Build history of the part. All positions in model axes, mm. A direction names the side the tool comes from. Coordinates: 2 decimals unless noted, no trailing zeros. Loops run counter-clockwise (first coordinate to the right, second up) from the corner with the lowest first, then second, coordinate; pieces in that order, holes last.
Item 1: Mould opens along Z. For faces 3 (the face through (0.66, 7.43, -14.985)), 4 (the face through (0, 2.5, 0)), 5 (the face through (1, 2.5, 17)) say: released by +Z, released by -Z, zero draft, split by the parting line, or undercut.
Item 2: Cut at C-C (y = -1). List the corners of the cut face in (x, z), and give its area (3 significant figures).
Item 3: Cut at B-B (x = 0). List the corners of the cut face in (y, z), and give its area (3 significant figures).
Item 4: 3-axis set-ups, long thin cutter, end or side, ignore diameter. For faces 1 (the face through (1, -2.5, -1)), 2 (the face through (-9.76, 7.43, -2.17)): which of +Z, -Z, +X, -X, +Y, -Y reach the whole face in a straight line?
Item 5: Flat gauge pins, fed straight in: pin 1 (3.5 mm diameter, centred on x = 0, z = -30, fed in from -Y); pin 2 (8 mm diameter, centred on y = -0.5, z = -2.5, fed in from -X); pin 3 (1 mm diameter, centred on y = 8.5, z = 12, fed in from -X); pin 4 (5 mm diameter, centred on y = 1.5, z = 5.5, fed in from -X). Where does each tip first touch, or does it go through?
Item 6: Cut at D-D (z = 30). List the corners of the cut face in (x, y), and give its area (3 significant figures).
Item 7: Cut at A-A (z = 0). List the corners of the cut face in (x, y).
Item 8: Drill centre lines: line 1 along X through (y, z) = (-0.1, 0); line 2 along X through (y, z) = (6.75, 0); line 3 along Z through (x, y) = (-1, 2). Where is each one in solid material? Low to high.
from build123d import *

# Parameters (mm, degrees)
SKETCH1_R           = 40
SKETCH1_R_2         = 2
BOSS_EXTRUDE1_DEPTH = 2.5
SKETCH2_R           = 15
SKETCH2_R_2         = 10
BOSS_EXTRUDE2_DEPTH = 10


with BuildPart() as part:
    # Sketch1 → Boss-Extrude1 (new, symmetric)
    with BuildSketch(Plane(origin=(0, 0, 0), x_dir=(1, 0, 0), z_dir=(0, 1, 0))):
        with Locations(Location((0, 0, 0), (0, 0, 270))):
            Circle(SKETCH1_R)
        with Locations(Location((0, 30, 0), (0, 0, 270))):
            Circle(SKETCH1_R_2, mode=Mode.SUBTRACT)
        with Locations(Location((30, 0, 0), (0, 0, 270))):
            Circle(SKETCH1_R_2, mode=Mode.SUBTRACT)
        with Locations(Location((0, -30, 0), (0, 0, 270))):
            Circle(SKETCH1_R_2, mode=Mode.SUBTRACT)
        with Locations(Location((-30, 0, 0), (0, 0, 270))):
            Circle(SKETCH1_R_2, mode=Mode.SUBTRACT)
    extrude(amount=BOSS_EXTRUDE1_DEPTH, both=True)

    # Sketch2 → Boss-Extrude2 (add)
    with BuildSketch(Plane(origin=(0, 2.5, 0), x_dir=(1, 0, 0), z_dir=(0, 1, 0))):
        with Locations(Location((0, 0, 0), (0, 0, 270))):
            Circle(SKETCH2_R)
        with Locations(Location((0, 0, 0), (0, 0, 270))):
            Circle(SKETCH2_R_2, mode=Mode.SUBTRACT)
    extrude(amount=BOSS_EXTRUDE2_DEPTH)


solid = part.part
Filled sheet:
1. face 3: split by the parting line
1. face 4: undercut
1. face 5: zero draft
2. outline: circle Ø80 at (0, 0); hole circle Ø4 at (-30, 0); hole circle Ø4 at (0, -30); hole circle Ø4 at (0, 30); hole circle Ø4 at (30, 0)
2. area: 4,980 mm2
3. outline: (-2.5, -40) - (2.5, -40) - (2.5, -32) - (-2.5, -32) - close; (-2.5, -28) - (2.5, -28) - (2.5, -15) - (12.5, -15) - (12.5, -10) - (2.5, -10) - (2.5, 10) - (12.5, 10) - (12.5, 15) - (2.5, 15) - (2.5, 28) - (-2.5, 28) - close; (-2.5, 32) - (2.5, 32) - (2.5, 40) - (-2.5, 40) - close
3. area: 460 mm2
4. face 1: +Z, -Z, +X, -X, -Y
4. face 2: +Y
5. pin 1: passes through
5. pin 2: stops at x = -40
5. pin 3: stops at x = -9.63
5. pin 4: stops at x = -39.89
6. outline: (-26.46, -2.5) - (-2, -2.5) - (-2, 2.5) - (-26.46, 2.5) - close; (2, -2.5) - (26.46, -2.5) - (26.46, 2.5) - (2, 2.5) - close
6. area: 245 mm2
7. outline: (-40, -2.5) - (-32, -2.5) - (-32, 2.5) - (-40, 2.5) - close; (-28, -2.5) - (28, -2.5) - (28, 2.5) - (15, 2.5) - (15, 12.5) - (10, 12.5) - (10, 2.5) - (-10, 2.5) - (-10, 12.5) - (-15, 12.5) - (-15, 2.5) - (-28, 2.5) - close; (32, -2.5) - (40, -2.5) - (40, 2.5) - (32, 2.5) - close
8. line 1: x = -40 to -32, -28 to 28, 32 to 40
8. line 2: x = -15 to -10, 10 to 15
8. line 3: z = -39.99 to -31.73, -28.27 to 28.27, 31.73 to 39.99
